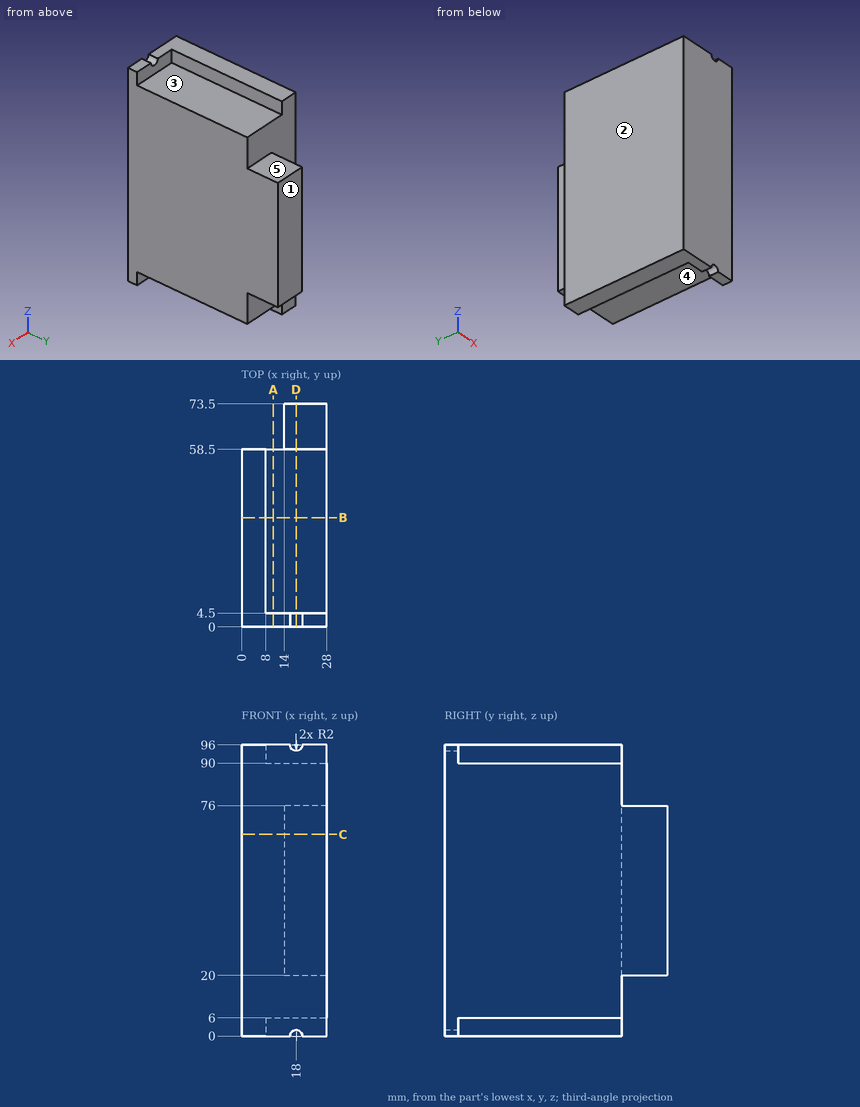
Geometry check sheet. Reference: drawing and pictorial views, mm from the part's lowest x, y, z. A direction names the side the tool comes from. Round coordinates to 2 decimals unless told otherwise and drop trailing zeros. Loops run counter-clockwise (first coordinate to the right, second up) from the corner with the lowest first, then second, coordinate; pieces in that order, holes last. Notation, with made-up numbers: (-21.75, 82.5) - (18.25, 82.5) arc R12 ccw to (18.25, 96.5) - close; hole circle Ø10 at (-13, 34). An arc over 180 degrees is marked (long way). Use a Markdown table: item, result.
Q1. Cross-section at A-A on x = 10.5. Record the cut outline in (y, z).
Solutions:
| item | result |
|---|---|
| outline | (0, 0) - (4.5, 0) - (4.5, 6) - (58.5, 6) - (58.5, 90) - (4.5, 90) - (4.5, 96) - (0, 96) - close |
Q2. Cross-section at B-B on y = 36. Record the cut outline in (x, z).
Solutions:
| item | result |
|---|---|
| outline | (0, 0) - (8, 0) - (8, 6) - (28, 6) - (28, 90) - (8, 90) - (8, 96) - (0, 96) - close |
Q3. Go/stop test with flat-tipped pins: P1, Ø3, axis at x = 8, z = 19, coming from the +Y side; P2, Ø15.5, axis at x = 22.5, y = 64, coming from the +Z side; P3, Ø11, axis at x = 19, y = 68, coming from the -Z side. Record where each tip stops, or that it passes through.
Solutions:
| item | result |
|---|---|
| P1 | stops at y = 58.5 |
| P2 | stops at z = 90 |
| P3 | stops at z = 20 |
Q4. Cross-section at C-C on z = 66.5. Record the cut outline in (x, y), plus the area to 3 significant figures.
Solutions:
| item | result |
|---|---|
| outline | (0, 0) - (28, 0) - (28, 73.5) - (14, 73.5) - (14, 58.5) - (0, 58.5) - close |
| area | 1,850 mm2 |
Q5. Access from +Z, -Z, +X, -X, +Y, -Y to the whole of each face (thin tool, end or side, straight path). Record for the marked faces 1, 2, 3, 4 and 5.
Solutions:
| item | result |
|---|---|
| face 1 | +Z, -Z, +X, -X, +Y |
| face 2 | +Z, -Z, -X, +Y, -Y |
| face 3 | +Z, +X, +Y |
| face 4 | -Z, +X, +Y |
| face 5 | +Z, +X, -X, +Y |
Q6. Material ranges on line 1 (Z direction, x = 14.25, y = 46.5); line 2 (Y direction, x = 8.75, z = 78.5); line 3 (X direction, y = 69.5, z = 31), recorded low to high.
Solutions:
| item | result |
|---|---|
| line 1 | z = 6 to 90 |
| line 2 | y = 0 to 58.5 |
| line 3 | x = 14 to 28 |
Q7. Cross-section at D-D on x = 18. Record the cut outline in (y, z).
Solutions:
| item | result |
|---|---|
| outline | (0, 2) - (4.5, 2) - (4.5, 6) - (58.5, 6) - (58.5, 20) - (73.5, 20) - (73.5, 76) - (58.5, 76) - (58.5, 90) - (4.5, 90) - (4.5, 94) - (0, 94) - close |
